from build123d import *

# Parameters (mm, degrees)
F0_W      = 50
F0_H      = 50
F0_R      = 2.75
F1_DEPTH  = 5
F2_R      = 20
F3_DEPTH  = 17
F7_R      = 7.5
F8_DEPTH  = 40.001
F9_R      = 2.5
F10_DEPTH = 25.001


with BuildPart() as f1:
    # F0 (on Front) → F1 (new body)
    with BuildSketch(Plane.XZ):
        with Locations((25, 25)):
            Rectangle(F0_W, F0_H)
        with Locations((5, 5)):
            Circle(F0_R, mode=Mode.SUBTRACT)
        with Locations((45, 5)):
            Circle(F0_R, mode=Mode.SUBTRACT)
        with Locations((5, 45)):
            Circle(F0_R, mode=Mode.SUBTRACT)
        with Locations((45, 45)):
            Circle(F0_R, mode=Mode.SUBTRACT)
    extrude(amount=F1_DEPTH)

    # F2 (on face) → F3 (join)
    with BuildSketch(Plane.XZ.offset(5)):
        with Locations((25, 25)):
            Circle(F2_R)
    extrude(amount=F3_DEPTH)

    # F5 (on offset) → F6 (revolve)
    with BuildSketch(Plane.XY.offset(25)):
        Polygon((12.5, -40), (17.5, -40), (17.5, -22), (5, -22), align=None)
    revolve(axis=Axis((25, -31, 25), (0, -1, 0)))

    # F7 (on face) → F8 (cut, through all)
    with BuildSketch(Plane(origin=(0, 0, 0), x_dir=(-1, 0, 0), z_dir=(0, 1, 0))):
        with Locations((-25, 25)):
            Circle(F7_R)
    extrude(amount=-F8_DEPTH, mode=Mode.SUBTRACT)

    # F9 (on offset) → F10 (cut, through all)
    with BuildSketch(Plane.XY.offset(25)):
        with Locations((25, -13.5)):
            Circle(F9_R)
    extrude(amount=-F10_DEPTH, mode=Mode.SUBTRACT)


solid = f1.part
Model file for the job. Use its own axes, mm. A direction names the side the tool comes from. Give positions to 0.01 mm unless a question says otherwise; leave off trailing zeros. Order: outer loops, then holes, each group sorted by start corner. A loop starts at its lowest first (then second) coordinate and runs counter-clockwise, first axis right, second up. Notation, with made-up numbers: (-3.5, 68) - (18.5, 68) arc R22 cw to (18.5, 81) - close; hole circle Ø2 at (44, 8). An arc over 180 degrees is marked (long way). Return JSON: item names as keys, results as strings.
1) Cut at C-C, the plane z = 43. Count the separate pieces of the cut face and the enclosed holes in it, plus the area to 3 significant figures.
Geometry says:
{"separate pieces": "3", "enclosed holes": "0", "area": "564 mm²"}
2) Pull direction X, two halves, no side cores. Call faces 1 (the flat face through (0, -2, 25)), 2 (the flat face through (25, -2, 0)), 3 (the cylindrical face through (4.642, -2.465, 47.727)): pulls with the +X half, pulls with the -X half, needs draft (parallel to the pull), parting line crosses it, or undercut.
Geometry says:
{"face 1": "pulls with the -X half", "face 2": "needs draft", "face 3": "undercut"}
3) Cut at A-A, the plane x = 25. Give the cut face in (y, z).
Geometry says:
{"outline": "(-40, 12.5) - (-22, 5) - (-16, 5) - (-16, 17.5) - (-40, 17.5) - close; (-40, 32.5) - (0, 32.5) - (0, 50) - (-5, 50) - (-5, 45) - (-22, 45) - (-40, 37.5) - close; (-11, 5) - (-5, 5) - (-5, 0) - (0, 0) - (0, 17.5) - (-11, 17.5) - close"}
4) 3-axis set-ups, long thin cutter, end or side, ignore diameter. For faces 4 (the cylindrical face through (23, -15, 12)), 5 (the cylindrical face through (42.253, -2.465, 5.121)), 6 (the flat face through (8, -5, 36)): which of +Z, -Z, +X, -X, +Y, -Y reach the whole face in a straight line?
Geometry says:
{"face 4": "-Z", "face 5": "+Y, -Y", "face 6": "-Y"}
5) Flat gauge pins, fed straight in: P1, Ø2, axis at x = 42, z = 34.5, coming from the +Y side; P2, Ø1, axis at x = 36.5, y = -19, coming from the +Z side; P3, Ø6, axis at x = 25, y = -13.5, coming from the +Z side; P4, Ø2, axis at y = -26.5, z = 25, coming from the -X side. Where does each tip first touch, or does it go through?
Geometry says:
{"P1": "y = 0", "P2": "z = 41.7", "P3": "z = 45", "P4": "x = 6.46"}
6) Cut at B-B, the plane y = -20.5. Give the cut face in (x, z).
Geometry says:
{"outline": "circle Ø40 at (25, 25); hole circle Ø15 at (25, 25)"}
7) Cut at D-D, the plane y = -13.5. Give the cut face in (x, z), plus the area to 3 significant figures.
Geometry says:
{"outline": "(22.5, 5.16) - (22.5, 17.93) arc R7.5 cw (long way) to (27.5, 17.93) - (27.5, 5.16) arc R20 ccw (long way) to start", "area": "1,020 mm²"}
8) Probe line 1 (Z direction, x = 45, y = -3.05); line 2 (X direction, y = -14.5, z = 25); line 3 (X direction, y = -3, z = 22.5). List the from-to ranges inside material, lowest first. Write a range as from..to.
Geometry says:
{"line 1": "0..2.25, 7.75..42.25, 47.75..50", "line 2": "5..17.5, 32.5..45", "line 3": "0..17.93, 32.07..50"}
